from build123d import *

# Parameters (mm, degrees)
SKETCH1_W           = 50.8
SKETCH1_H           = 342.9
BOSS_EXTRUDE1_DEPTH = 25.4
SHELL1_T            = -3.175
SKETCH2_R           = 2.4892
CUT_EXTRUDE1_DEPTH  = 51.8
SKETCH3_R           = 2.4892
CUT_EXTRUDE2_DEPTH  = 26.4
CUT_EXTRUDE3_REACH  = 27.4
SKETCH4_R           = 2.4892
SKETCH6_R           = 2.4892
CUT_EXTRUDE5_DEPTH  = 26.4


with BuildPart() as part:
    # Sketch1 → Boss-Extrude1 (new body)
    with BuildSketch(Plane(origin=(0, 0, 0), x_dir=(1, 0, 0), z_dir=(0, 1, 0))):
        with Locations((25.4, 171.45)):
            Rectangle(SKETCH1_W, SKETCH1_H)
    extrude(amount=BOSS_EXTRUDE1_DEPTH)

    # Shell1
    shell1_openings = [part.faces().sort_by_distance(p)[0] for p in [
        (25.4, 12.7, -342.9),
        (25.4, 12.7, 0),
    ]]
    offset(amount=SHELL1_T, openings=shell1_openings, kind=Kind.INTERSECTION)

    # Sketch2 → Cut-Extrude1 (cut, through all)
    with BuildSketch(Plane.ZY):
        with Locations((-12.7, 12.7)):
            Circle(SKETCH2_R)
        with Locations((-38.1, 12.7)):
            Circle(SKETCH2_R)
        with Locations((-63.5, 12.7)):
            Circle(SKETCH2_R)
        with Locations((-88.9, 12.7)):
            Circle(SKETCH2_R)
        with Locations((-114.3, 12.7)):
            Circle(SKETCH2_R)
        with Locations((-139.7, 12.7)):
            Circle(SKETCH2_R)
        with Locations((-165.1, 12.7)):
            Circle(SKETCH2_R)
        with Locations((-190.5, 12.7)):
            Circle(SKETCH2_R)
        with Locations((-215.9, 12.7)):
            Circle(SKETCH2_R)
        with Locations((-241.3, 12.7)):
            Circle(SKETCH2_R)
        with Locations((-266.7, 12.7)):
            Circle(SKETCH2_R)
    extrude(amount=-CUT_EXTRUDE1_DEPTH, mode=Mode.SUBTRACT)

    # Sketch3 → Cut-Extrude2 (cut, through all)
    with BuildSketch(Plane(origin=(0, 25.4, 0), x_dir=(1, 0, 0), z_dir=(0, 1, 0))):
        with Locations((12.7, 293.424634479)):
            Circle(SKETCH3_R)
        with Locations((38.1, 293.424634479)):
            Circle(SKETCH3_R)
        with Locations((38.1, 306.124634479)):
            Circle(SKETCH3_R)
        with Locations((12.7, 306.124634479)):
            Circle(SKETCH3_R)
        with Locations((12.7, 318.824634479)):
            Circle(SKETCH3_R)
        with Locations((38.1, 318.824634479)):
            Circle(SKETCH3_R)
        with Locations((38.1, 331.524634479)):
            Circle(SKETCH3_R)
        with Locations((12.7, 331.524634479)):
            Circle(SKETCH3_R)
    extrude(amount=-CUT_EXTRUDE2_DEPTH, mode=Mode.SUBTRACT)

    # Sketch4 → Cut-Extrude3 (cut, up to next)
    with BuildSketch(Plane.XZ, mode=Mode.PRIVATE) as cut_extrude3_sk1:
        with Locations((38.1, -12.7)):
            Circle(SKETCH4_R)
    cut_extrude3_tool1 = extrude(cut_extrude3_sk1.sketch, amount=-CUT_EXTRUDE3_REACH, mode=Mode.PRIVATE) & part.part
    add(cut_extrude3_tool1.solids().sort_by_distance((38.1, 0, -12.7))[0], mode=Mode.SUBTRACT)
    # Sketch4 → Cut-Extrude3 (cut, up to next)
    with BuildSketch(Plane.XZ, mode=Mode.PRIVATE) as cut_extrude3_sk2:
        with Locations((12.7, -12.7)):
            Circle(SKETCH4_R)
    cut_extrude3_tool2 = extrude(cut_extrude3_sk2.sketch, amount=-CUT_EXTRUDE3_REACH, mode=Mode.PRIVATE) & part.part
    add(cut_extrude3_tool2.solids().sort_by_distance((12.7, 0, -12.7))[0], mode=Mode.SUBTRACT)
    # Sketch4 → Cut-Extrude3 (cut, up to next)
    with BuildSketch(Plane.XZ, mode=Mode.PRIVATE) as cut_extrude3_sk3:
        with Locations((12.7, -25.4)):
            Circle(SKETCH4_R)
    cut_extrude3_tool3 = extrude(cut_extrude3_sk3.sketch, amount=-CUT_EXTRUDE3_REACH, mode=Mode.PRIVATE) & part.part
    add(cut_extrude3_tool3.solids().sort_by_distance((12.7, 0, -25.4))[0], mode=Mode.SUBTRACT)
    # Sketch4 → Cut-Extrude3 (cut, up to next)
    with BuildSketch(Plane.XZ, mode=Mode.PRIVATE) as cut_extrude3_sk4:
        with Locations((38.1, -25.4)):
            Circle(SKETCH4_R)
    cut_extrude3_tool4 = extrude(cut_extrude3_sk4.sketch, amount=-CUT_EXTRUDE3_REACH, mode=Mode.PRIVATE) & part.part
    add(cut_extrude3_tool4.solids().sort_by_distance((38.1, 0, -25.4))[0], mode=Mode.SUBTRACT)
    # Sketch4 → Cut-Extrude3 (cut, up to next)
    with BuildSketch(Plane.XZ, mode=Mode.PRIVATE) as cut_extrude3_sk5:
        with Locations((38.1, -38.1)):
            Circle(SKETCH4_R)
    cut_extrude3_tool5 = extrude(cut_extrude3_sk5.sketch, amount=-CUT_EXTRUDE3_REACH, mode=Mode.PRIVATE) & part.part
    add(cut_extrude3_tool5.solids().sort_by_distance((38.1, 0, -38.1))[0], mode=Mode.SUBTRACT)
    # Sketch4 → Cut-Extrude3 (cut, up to next)
    with BuildSketch(Plane.XZ, mode=Mode.PRIVATE) as cut_extrude3_sk6:
        with Locations((12.7, -38.1)):
            Circle(SKETCH4_R)
    cut_extrude3_tool6 = extrude(cut_extrude3_sk6.sketch, amount=-CUT_EXTRUDE3_REACH, mode=Mode.PRIVATE) & part.part
    add(cut_extrude3_tool6.solids().sort_by_distance((12.7, 0, -38.1))[0], mode=Mode.SUBTRACT)
    # Sketch4 → Cut-Extrude3 (cut, up to next)
    with BuildSketch(Plane.XZ, mode=Mode.PRIVATE) as cut_extrude3_sk7:
        with Locations((12.7, -50.8)):
            Circle(SKETCH4_R)
    cut_extrude3_tool7 = extrude(cut_extrude3_sk7.sketch, amount=-CUT_EXTRUDE3_REACH, mode=Mode.PRIVATE) & part.part
    add(cut_extrude3_tool7.solids().sort_by_distance((12.7, 0, -50.8))[0], mode=Mode.SUBTRACT)
    # Sketch4 → Cut-Extrude3 (cut, up to next)
    with BuildSketch(Plane.XZ, mode=Mode.PRIVATE) as cut_extrude3_sk8:
        with Locations((38.1, -50.8)):
            Circle(SKETCH4_R)
    cut_extrude3_tool8 = extrude(cut_extrude3_sk8.sketch, amount=-CUT_EXTRUDE3_REACH, mode=Mode.PRIVATE) & part.part
    add(cut_extrude3_tool8.solids().sort_by_distance((38.1, 0, -50.8))[0], mode=Mode.SUBTRACT)
    # Sketch4 → Cut-Extrude3 (cut, up to next)
    with BuildSketch(Plane.XZ, mode=Mode.PRIVATE) as cut_extrude3_sk9:
        with Locations((38.1, -63.5)):
            Circle(SKETCH4_R)
    cut_extrude3_tool9 = extrude(cut_extrude3_sk9.sketch, amount=-CUT_EXTRUDE3_REACH, mode=Mode.PRIVATE) & part.part
    add(cut_extrude3_tool9.solids().sort_by_distance((38.1, 0, -63.5))[0], mode=Mode.SUBTRACT)
    # Sketch4 → Cut-Extrude3 (cut, up to next)
    with BuildSketch(Plane.XZ, mode=Mode.PRIVATE) as cut_extrude3_sk10:
        with Locations((12.7, -63.5)):
            Circle(SKETCH4_R)
    cut_extrude3_tool10 = extrude(cut_extrude3_sk10.sketch, amount=-CUT_EXTRUDE3_REACH, mode=Mode.PRIVATE) & part.part
    add(cut_extrude3_tool10.solids().sort_by_distance((12.7, 0, -63.5))[0], mode=Mode.SUBTRACT)

    # Sketch6 → Cut-Extrude5 (cut, through all)
    with BuildSketch(Plane.XZ):
        Polygon((0, -307.473161113), (0, -342.9), (24.806139644, -342.9), align=None)
        with Locations((12.7, -331.524634479)):
            Circle(SKETCH6_R, mode=Mode.SUBTRACT)
    extrude(amount=-CUT_EXTRUDE5_DEPTH, mode=Mode.SUBTRACT)


solid = part.part
Can you work these out from the model? Positions are in its coordinate system, mm. A direction names the side the tool comes from. Give positions to 0.01 mm unless a question says otherwise; leave off trailing zeros. Loops run counter-clockwise (first coordinate to the right, second up) from the corner with the lowest first, then second, coordinate; pieces in that order, holes last. Notation, with made-up numbers: (35, 86.25) -> (45, 86.25) arc R28 ccw to (45, 108.25) -> close; hole circle Ø8 at (23.25, 88.25). An arc over 180 degrees is marked (long way). Use one line per item in the form item = value.
1) If we section it at A-A (x = 32): Please give me the cut outline in (y, z) (3 decimals).
Answers:
outline = (0, -342.9) -> (3.175, -342.9) -> (3.175, 0) -> (0, 0) -> close; (22.225, -342.9) -> (25.4, -342.9) -> (25.4, 0) -> (22.225, 0) -> close
2) I need wall thicknesses on line 1 along X through (y, z) = (14, -260) (3 decimals); line 2 along Y through (x, z) = (27.5, -197) (3 decimals); line 3 along X through (y, z) = (10.5, -314.5) (3 decimals). Which ranges of each line are inside material? Lowest first, please.
Answers:
line_1 = 0 to 3.175, 47.625 to 50.8
line_2 = 0 to 3.175, 22.225 to 25.4
line_3 = 47.625 to 50.8
3) We'd pull the mould along X, two halves only. Please class faces 1 (the face through (47.625, 13, -169)), 2 (the face through (25, 25.4, -174)), 3 (the face through (9.705, 22.989, -321.333)), 4 (the face through (50.8, 13, -169)): released by +X, released by -X, zero draft, split by the parting line, or undercut.
Answers:
face_1 = undercut
face_2 = zero draft
face_3 = released by -X
face_4 = released by +X
4) For faces 5 (the face through (25, 2, 0)), 6 (the face through (25, 3.175, -174)), which set-ups out of +Z, -Z, +X, -X, +Y, -Y let a thin tool reach every point of the face, with its end or its side?
Answers:
face_5 = +Z, +X, -X, +Y, -Y
face_6 = +Z, -Z
5) Will this pin go through, and if not, where does the flat tip stop? pin 1 (4.5 mm diameter, centred on y = 12.7, z = -12.7, fed in from +X).
Answers:
pin_1 = through
6) If we section it at B-B (z = -152): Please give me the cut outline in (x, y) (3 decimals), plus the area to 3 significant figures.
Answers:
outline = (0, 0) -> (50.8, 0) -> (50.8, 25.4) -> (0, 25.4) -> close; hole (3.175, 3.175) -> (47.625, 3.175) -> (47.625, 22.225) -> (3.175, 22.225) -> close
area = 444 mm²
